```python
from build123d import *

# Parameters (mm, degrees)
STOCK_BUMBLE_START            = -47.625
STOCK_BUMBLE_BYTE_1_OUTLINE_R = 2.7051
STOCK_BUMBLE_BYTE_1_DEPTH     = 9.525
FILLET1_R                     = 2.54
FILLET2_R                     = 1.27
FILLET3_R                     = 1.27
FILLET4_R                     = 25.4


# Read off the part's stored shape, not the designer's step: Stock-Bumble Byte-1
with BuildPart() as part:
    # Stock-Bumble Byte-1 outline → Stock-Bumble Byte-1 (new body)
    with BuildSketch(Plane.YZ.offset(STOCK_BUMBLE_START)):
        Polygon((21.9075, 120.65), (11.1125, 34.7472), (11.1125, 27.1272), (39.6875, 27.1272), (39.6875, 34.7472), (28.8925, 120.65), (30.766729518, 120.65), (25.4, 152.4), (20.033270482, 120.65), align=None)
        with Locations((15.875, 33.4772)):
            Circle(STOCK_BUMBLE_BYTE_1_OUTLINE_R, mode=Mode.SUBTRACT)
        with Locations((25.4, 37.143795847)):
            Circle(STOCK_BUMBLE_BYTE_1_OUTLINE_R, mode=Mode.SUBTRACT)
        with Locations((34.925, 33.4772)):
            Circle(STOCK_BUMBLE_BYTE_1_OUTLINE_R, mode=Mode.SUBTRACT)
        with BuildLine():
            ThreePointArc((32.573016025, 40.433269228), (25.4, 41.944395847), (18.226983975, 40.433269228))
            Line((18.226983975, 40.433269228), (25.4, 97.513599106))
            Line((25.4, 97.513599106), (32.573016025, 40.433269228))
        make_face(mode=Mode.SUBTRACT)
    extrude(amount=STOCK_BUMBLE_BYTE_1_DEPTH)

    # Fillet1
    fillet1_edges = [part.edges().sort_by_distance(p)[0] for p in [
        (-42.8625, 11.1125, 27.1272),
        (-42.8625, 39.6875, 27.1272),
    ]]
    fillet(fillet1_edges, radius=FILLET1_R)

    # Fillet2
    fillet2_edges = [part.edges().sort_by_distance(p)[0] for p in [
        (-42.8625, 18.226983975, 40.433269228),
        (-42.8625, 32.573016025, 40.433269228),
        (-42.8625, 25.4, 97.513599106),
    ]]
    fillet(fillet2_edges, radius=FILLET2_R)

    # Fillet3
    fillet3_edges = [part.edges().sort_by_distance(p)[0] for p in [
        (-42.8625, 28.8925, 120.65),
        (-42.8625, 21.9075, 120.65),
    ]]
    fillet(fillet3_edges, radius=FILLET3_R)

    # Fillet4
    fillet4_edges = [part.edges().sort_by_distance(p)[0] for p in [
        (-42.8625, 11.1125, 34.7472),
        (-42.8625, 39.6875, 34.7472),
    ]]
    fillet(fillet4_edges, radius=FILLET4_R)


solid = part.part
```
Work out the finished part from the listing and answer in its coordinate system (mm). A direction names the side the tool comes from. Round coordinates to 2 decimals unless told otherwise and drop trailing zeros. Order: outer loops, then holes, each group sorted by start corner. A loop starts at its lowest first (then second) coordinate and runs counter-clockwise, first axis right, second up.
Q1. A cutting plane is placed at A-A, the plane z = 72. Determine the outline of the cut face in (x, y) (3 decimals), then the cut area to 3 significant figures.
Solution:
outline: (-47.625, 15.794) - (-38.1, 15.794) - (-38.1, 22.194) - (-47.625, 22.194) - close; (-47.625, 28.606) - (-38.1, 28.606) - (-38.1, 35.006) - (-47.625, 35.006) - close
area: 122 mm2
Q2. Given pin 1 Ø1 at (x, z) = (-40, 129) entering from -Y; pin 2 Ø5 at (x, z) = (-45, 50) entering from -Y; pin 3 Ø5 at (y, z) = (34.92, 33.48) entering from -X; pin 4 Ø2 at (x, z) = (-42.5, 44) entering from +Y, each flat-ended and moving along its own axis, determine where each tip first touches the part or whether it passes through.
Solution:
pin 1: stops at y = 21.36
pin 2: stops at y = 12.72
pin 3: passes through
pin 4: stops at y = 38.65
Q3. The mould has two halves that part along Z. Classify faces 4 (the cylindrical face through (-42.8, 38.92, 27.85)), 5 (the cylindrical face through (-42.929, 17.123, 31.077)), 6 (the flat face through (-42.93, 28.12, 136.3)): pulls with the +Z half, pulls with the -Z half, needs draft (parallel to the pull), parting line crosses it, or undercut.
Solution:
face 4: pulls with the -Z half
face 5: undercut
face 6: pulls with the +Z half
Q4. A tool of negligible diameter and unlimited length cuts with its end or side. For faces 1 (the flat face through (-42.929, 29.446, 65.316)), 2 (the flat face through (-43, 39.688, 31)), 3 (the flat face through (-42.9, 16.6, 78.4)), from which of +Z, -Z, +X, -X, +Y, -Y can it reach the whole face along a straight path? Write none if from no direction.
Solution:
face 1: +X, -X
face 2: +Z, -Z, +X, -X, +Y
face 3: +X, -X, -Y
Q5. Find the intervals of material crossed by line 1 along Y through (x, z) = (-44.75, 35); line 2 along Y through (x, z) = (-41, 61); line 3 along Y through (x, z) = (-43.25, 65.5), in increasing order.
Solution:
line 1: y = 11.18 to 13.64, 18.11 to 23.75, 27.05 to 32.69, 37.16 to 39.62
line 2: y = 14.41 to 20.81, 29.99 to 36.39
line 3: y = 14.98 to 21.38, 29.42 to 35.82
Q6. A cutting plane is placed at C-C, the plane z = 124.5. Determine the outline of the cut face in (x, y) (3 decimals), then the cut area to 3 significant figures.
Solution:
outline: (-47.625, 20.684) - (-38.1, 20.684) - (-38.1, 30.116) - (-47.625, 30.116) - close
area: 89.8 mm2
Q7. A cutting plane is placed at B-B, the plane x = -43.75. Count the separate pieces of the cut face and the enclosed holes in it, then the cut area to 3 significant figures.
Solution:
separate pieces: 1
enclosed holes: 4
area: 1,460 mm2
